Build history of the part. All positions in model axes, mm. Face numbers are marked on the shaded views. A direction names the side the tool comes from. Coordinates: 2 decimals unless noted, no trailing zeros. Write each loop counter-clockwise with the first axis right and the second up, starting at its lowest first coordinate (ties: lowest second). Pieces come first, ordered by that corner, then holes.
Autodesk Fusion 360 part; units mm, degrees
sketch "Sketch1" plane through (0, 0, 0) normal (0, 0, 1) x (1, 0, 0)
  line L0 (12, -18) -> (-12, -18)
  line L1 (-12, -18) -> (-12, 18)
  line L2 (-12, 18) -> (12, 18)
  line L3 (12, 18) -> (12, -18)
  line L4 (12, -18) -> (-12, 18) construction
  line L5 (-12, -18) -> (12, 18) construction
  dimension "d1" = 36
  dimension "d2" = 24
extrude "Extrude1" add sketch "Sketch1" along normal blind 24
chamfer "Chamfer1" distance 4 angle 45 4 edges at (12, -18, 12) (12, 18, 12) (-12, -18, 12) (-12, 18, 12)
sketch "Sketch2" plane through (0, 0, 24) normal (0, 0, 1) x (-1, 0, 0)
  line L0 (8, -18) -> (12, -14)
  line L1 (12, -14) -> (12, 14)
  line L2 (12, 14) -> (8, 18)
  line L3 (8, 18) -> (-8, 18)
  line L4 (-8, 18) -> (-12, 14)
  line L5 (-12, 14) -> (-12, -14)
  line L6 (-12, -14) -> (-8, -18)
  line L7 (-8, -18) -> (8, -18)
  circle A0 centre (0, -9) radius 9
  circle A1 centre (0, -9) radius 6 construction
  line L8 (0, 0) -> (0, -18) construction
  circle A2 centre (0, -15) radius 1.75
  circle A3 centre (6, -9) radius 1.75
  circle A4 centre (0, -3) radius 1.75
  circle A5 centre (-6, -9) radius 1.75
  dimension "d6" = 18
  dimension "d7" = 12
  dimension "d8" = 3.5
  dimension "d10" = 360
extrude "Extrude2" add sketch "Sketch2" along normal blind 3 contours A0
sketch "Sketch3" plane through (0, -18, 0) normal (0, -1, 0) x (1, 0, 0)
  line L0 (-8, 24) -> (-8, 0)
  line L1 (-8, 0) -> (8, 0)
  line L2 (8, 0) -> (8, 24)
  line L3 (8, 24) -> (-8, 24)
  line L4 (-12, 0) -> (12, 0)
  line L5 (12, 0) -> (12, 24)
  line L6 (12, 24) -> (-12, 24)
  line L7 (-12, 24) -> (-12, 0)
  line L8 (-12, 21) -> (12, 21)
  line L9 (-12, 3) -> (12, 3)
  point P0 (-12, 24)
  point P1 (12, 24)
  point P2 (12, 0)
  point P3 (-12, 0)
  dimension "d13" = 3
  dimension "d14" = 3
extrude "Extrude3" cut sketch "Sketch3" against normal blind 4.5 contours L0 L2 L8 L9 | L0 L7 L8 L9 | L2 L5 L8 L9
sketch "Sketch5" plane through (0, 0, 24) normal (0, 0, 1) x (-1, 0, 0)
  line L0 (8, -18) -> (12, -14)
  line L1 (12, -14) -> (12, 14)
  line L2 (12, 14) -> (8, 18)
  line L3 (8, 18) -> (-8, 18)
  line L4 (-8, 18) -> (-12, 14)
  line L5 (-12, 14) -> (-12, -14)
  line L6 (-12, -14) -> (-8, -18)
  line L7 (-8, -18) -> (0, -18)
  circle A0 centre (0, -9) radius 9
  line L8 (0, -18) -> (8, -18)
  line L9 (12, 14) -> (-12, 14) construction
  line L10 (0, 14) -> (0, 18) construction
  line L11 (10, 16) -> (-10, 16) construction
  circle A1 centre (0, 16) radius 1.7
  circle A2 centre (-6, 16) radius 1.7
  circle A3 centre (6, 16) radius 1.7
  dimension "d17" = 3.4
  dimension "d20" = 6
  dimension "d21" = 0
extrude "Extrude4" cut sketch "Sketch5" along normal through all contours A1 | A2 | A3
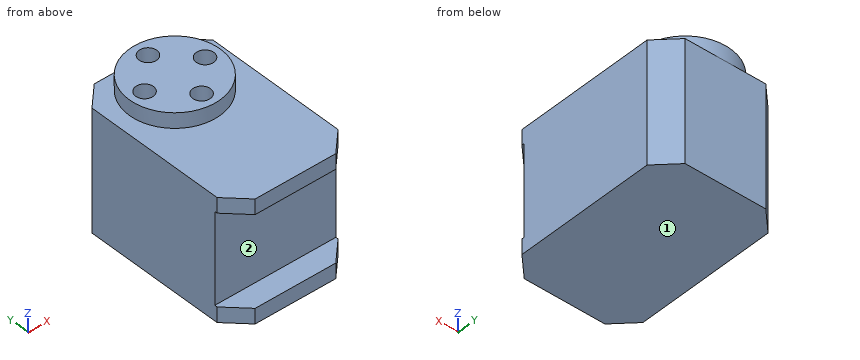
1. Saw through at C-C on z = 16. List the corners of the cut face in (x, y), plus the area to 3 significant figures.
Computed values:
outline: (-12, -13.5) - (12, -13.5) - (12, 14) - (8, 18) - (-8, 18) - (-12, 14) - close
area: 740 mm2
2. Saw through at D-D on y = 9. List the corners of the cut face in (x, z), plus the area to 3 significant figures.
Computed values:
outline: (-12, 0) - (12, 0) - (12, 24) - (9, 24) - (9, 27) - (7.75, 27) - (7.75, 24) - (4.25, 24) - (4.25, 27) - (-4.25, 27) - (-4.25, 24) - (-7.75, 24) - (-7.75, 27) - (-9, 27) - (-9, 24) - (-12, 24) - close
area: 609 mm2
3. Saw through at A-A on y = -15. List the corners of the cut face in (x, z), plus the area to 3 significant figures.
Computed values:
outline: (-11, 0) - (11, 0) - (11, 3) - (-11, 3) - close; (-11, 21) - (11, 21) - (11, 24) - (-11, 24) - close
area: 132 mm2
4. Saw through at B-B on x = 4.75. List the corners of the cut face in (y, z), plus the area to 3 significant figures.
Computed values:
outline: (-18, 0) - (18, 0) - (18, 24) - (16.64, 24) - (16.64, 27) - (10.22, 27) - (10.22, 24) - (7.78, 24) - (7.78, 27) - (1.36, 27) - (1.36, 24) - (-18, 24) - (-18, 21) - (-13.5, 21) - (-13.5, 3) - (-18, 3) - close
area: 822 mm2
5. 3-axis set-ups, long thin cutter, end or side, ignore diameter. For the marked faces 1 and 2: which of +Z, -Z, +X, -X, +Y, -Y reach the whole face in a straight line?
Computed values:
face 1: -Z, +X, -X, +Y, -Y
face 2: +X, -X, -Y
6. Probe line 1 along Y through (x, z) = (0, 24.95); line 2 along X through (y, z) = (9, 25.15); line 3 along Z through (x, y) = (3, -9). List the from-to ranges inside material, lowest first.
Computed values:
line 1: y = 0 to 1.25, 4.75 to 13.25, 16.75 to 18
line 2: x = -9 to -7.75, -4.25 to 4.25, 7.75 to 9
line 3: z = 0 to 24
7. Flat gauge pin, fed straight in: pin 1 (3.5 mm diameter, centred on x = 2.5, y = -16.5, fed in from +Z). Where does the tip first touch, or does it go through?
Computed values:
pin 1: stops at z = 24
